```python
from build123d import *

# Parameters (mm, degrees)
BOSS_EXTRUDE1_DEPTH     = 5
SKETCH2_R               = 11
CUT_EXTRUDE1_DEPTH      = 6
CUT_EXTRUDE1_DEPTH_BACK = 6


with BuildPart() as part:
    # Sketch1 → Boss-Extrude1 (new body, symmetric)
    with BuildSketch(Plane.XY):
        Polygon((350, 232.421392473), (-350, 232.421392473), (-350, -67.578607527), (-65, -67.578607527), (-55, -57.578607527), (-55, 81.421392473), (55, 81.421392473), (55, -57.578607527), (65, -67.578607527), (350, -67.578607527), align=None)
    extrude(amount=BOSS_EXTRUDE1_DEPTH, both=True)

    # Sketch2 → Cut-Extrude1 (cut, two sides)
    with BuildSketch(Plane.XY) as cut_extrude1_sk:
        with Locations((0, 172.421392473)):
            Circle(SKETCH2_R)
    extrude(amount=CUT_EXTRUDE1_DEPTH, mode=Mode.SUBTRACT)
    extrude(cut_extrude1_sk.sketch, amount=-CUT_EXTRUDE1_DEPTH_BACK, mode=Mode.SUBTRACT)


solid = part.part
```
Here's how the part is built. I have some questions about the finished solid (model axes, mm). Round coordinates to 2 decimals unless told otherwise and drop trailing zeros. Write each loop counter-clockwise with the first axis right and the second up, starting at its lowest first coordinate (ties: lowest second). Pieces come first, ordered by that corner, then holes.
Q1. If we section it at C-C on z = 0.75: Write out the boundary of the cut face in (x, y), plus the area to 3 significant figures.
Q2. Will this pin go through, and if not, where does the flat tip stop? P1, Ø5, axis at x = 0, z = -1, coming from the -Y side.
Q3. If we section it at A-A on y = 26: Write out the boundary of the cut face in (x, z).
Q4. Please list where these lines run through material, in increasing order: probe 1 along X at (y, z) = (-27.5, -3); probe 2 along Y at (x, z) = (0, 2.75).
Q5. If we mould it in two halves opening along Y, with no side actions, what happens to faces 1 (the flat face through (-5, 85, 5)), 2 (the cylindrical face through (-2.38, 161.68, 0.07))? For each: +Y half, -Y half, draft (parallel to the pull), parting line (faces both ways), or undercut.
Q6. If we section it at B-B on x = 0: Write out the boundary of the cut face in (y, z), plus the area to 3 significant figures.
Answer below:
1. outline: (-350, -67.58) - (-65, -67.58) - (-55, -57.58) - (-55, 81.42) - (55, 81.42) - (55, -57.58) - (65, -67.58) - (350, -67.58) - (350, 232.42) - (-350, 232.42) - close; hole circle Ø22 at (0, 172.42)
1. area: 193,000 mm2
2. P1: stops at y = 81.42
3. outline: (-350, -5) - (-55, -5) - (-55, 5) - (-350, 5) - close; (55, -5) - (350, -5) - (350, 5) - (55, 5) - close
4. probe 1: x = -350 to -55, 55 to 350
4. probe 2: y = 81.42 to 161.42, 183.42 to 232.42
5. face 1: draft
5. face 2: undercut
6. outline: (81.42, -5) - (161.42, -5) - (161.42, 5) - (81.42, 5) - close; (183.42, -5) - (232.42, -5) - (232.42, 5) - (183.42, 5) - close
6. area: 1,290 mm2
